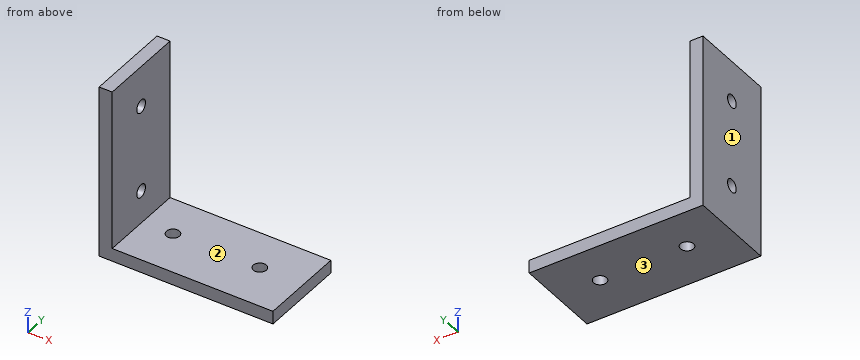
```python
from build123d import *

# Parameters (mm, degrees)
ESQUISSE1_W             = 40
ESQUISSE1_H             = 20
BOSS_EXTRU_1_DEPTH      = 3
ESQUISSE2_R             = 1.5
ENL_V_MAT_EXTRU_1_DEPTH = 3
ESQUISSE3_W             = 3
ESQUISSE3_H             = 20
BOSS_EXTRU_2_DEPTH      = 37
ESQUISSE4_R             = 1.5
ENL_V_MAT_EXTRU_2_DEPTH = 3


with BuildPart() as part:
    # Esquisse1 → Boss.-Extru.1 (new body)
    with BuildSketch(Plane.XY):
        with Locations((20, 10)):
            Rectangle(ESQUISSE1_W, ESQUISSE1_H)
    extrude(amount=BOSS_EXTRU_1_DEPTH)

    # Esquisse2 → Enlèv. mat.-Extru.1 (cut)
    with BuildSketch(Plane.XY.offset(3)):
        with Locations((10, 10.5)):
            Circle(ESQUISSE2_R)
        with Locations((30, 10.5)):
            Circle(ESQUISSE2_R)
    extrude(amount=-ENL_V_MAT_EXTRU_1_DEPTH, mode=Mode.SUBTRACT)

    # Esquisse3 → Boss.-Extru.2 (add)
    with BuildSketch(Plane.XY.offset(3)):
        with Locations((1.5, 10)):
            Rectangle(ESQUISSE3_W, ESQUISSE3_H)
    extrude(amount=BOSS_EXTRU_2_DEPTH)

    # Esquisse4 → Enlèv. mat.-Extru.2 (cut)
    with BuildSketch(Plane.ZY):
        with Locations((10.6, 10)):
            Circle(ESQUISSE4_R)
        with Locations((30.6, 10)):
            Circle(ESQUISSE4_R)
    extrude(amount=-ENL_V_MAT_EXTRU_2_DEPTH, mode=Mode.SUBTRACT)


solid = part.part
```
Can you work these out from the model? Positions are in its coordinate system, mm. Face numbers are marked on the shaded views. Give positions to 0.01 mm unless a question says otherwise; leave off trailing zeros. Write each loop counter-clockwise with the first axis right and the second up, starting at its lowest first coordinate (ties: lowest second). Pieces come first, ordered by that corner, then holes. Notation, with made-up numbers: (11, 63) - (50, 63) arc R25 cw to (50, 95) - close; hole circle Ø3 at (-30, 69). An arc over 180 degrees is marked (long way). Write item = value, one per line. Start each with the question number.
1. Imagine slicing it at B-B (x = 30). Please give me the cut outline in (y, z), and give its area (3 significant figures).
2. Imagine slicing it at C-C (y = 10.5). Please give me the cut outline in (x, z).
3. Thinking about a two-plate mould opening in Z: for the marked faces 1, 2 and 3, which applies, released by +Z, released by -Z, zero draft, split by the parting line, or undercut?
4. Please list where these lines run through material, in increasing order: line 1 (Y direction, x = 30, z = 2.1); line 2 (Y direction, x = 1.1, z = 30.6); line 3 (Z direction, x = 38.5, y = 9).
5. For pin 1 (2 mm diameter, centred on y = 2, z = 9.5, fed in from +X); pin 2 (2.5 mm diameter, centred on y = 10, z = 30.6, fed in from +X); pin 3 (4 mm diameter, centred on x = 30, y = 10.5, fed in from +Z), each with a flat end and sliding along its axis, tell me the tip position at first contact or that it passes through.
6. Imagine slicing it at D-D (z = 20.5). Please give me the cut outline in (x, y), and give its area (3 significant figures).
7. Imagine slicing it at A-A (z = 30.6). Please give me the cut outline in (x, y).
Worked answers:
q1.outline = (0, 0) - (9, 0) - (9, 3) - (0, 3) - close; (12, 0) - (20, 0) - (20, 3) - (12, 3) - close
q1.area = 51.0 mm2
q2.outline = (0, 0) - (8.5, 0) - (8.5, 3) - (3, 3) - (3, 9.19) - (0, 9.19) - close; (0, 12.01) - (3, 12.01) - (3, 29.19) - (0, 29.19) - close; (0, 32.01) - (3, 32.01) - (3, 40) - (0, 40) - close; (11.5, 0) - (28.5, 0) - (28.5, 3) - (11.5, 3) - close; (31.5, 0) - (40, 0) - (40, 3) - (31.5, 3) - close
q3.face_1 = zero draft
q3.face_2 = released by +Z
q3.face_3 = released by -Z
q4.line_1 = 0 to 9, 12 to 20
q4.line_2 = 0 to 8.5, 11.5 to 20
q4.line_3 = 0 to 3
q5.pin_1 = 3
q5.pin_2 = through
q5.pin_3 = 3
q6.outline = (0, 0) - (3, 0) - (3, 20) - (0, 20) - close
q6.area = 60.0 mm2
q7.outline = (0, 0) - (3, 0) - (3, 8.5) - (0, 8.5) - close; (0, 11.5) - (3, 11.5) - (3, 20) - (0, 20) - close
